Could you check a few things on this model? Use its own coordinates, in mm. A direction names the side the tool comes from. Give positions to 0.01 mm unless a question says otherwise; leave off trailing zeros. Loops run counter-clockwise (first coordinate to the right, second up) from the corner with the lowest first, then second, coordinate; pieces in that order, holes last. Notation, with made-up numbers: (-1, 68) - (48, 68) arc R21 cw to (48, 73) - close; hole circle Ø4 at (-25, 70.25). An arc over 180 degrees is marked (long way). Answer in a Markdown table with one row per item. Add a question column.
```python
from build123d import *

# Parameters (mm, degrees)
SKETCH1_W           = 70
SKETCH1_H           = 60
SKETCH1_R           = 1.5875
SKETCH1_R_2         = 4.499999999
BOSS_EXTRUDE1_DEPTH = 10


with BuildPart() as part:
    # Sketch1 → Boss-Extrude1 (new body)
    with BuildSketch(Plane(origin=(0, 0, 0), x_dir=(0, 0, -1), z_dir=(1, 0, 0))):
        with Locations((3.813160791, 27.897530874)):
            Rectangle(SKETCH1_W, SKETCH1_H)
        with Locations((-16.186839209, 52.897530874)):
            Circle(SKETCH1_R, mode=Mode.SUBTRACT)
        with Locations((-16.186839209, 2.897530874)):
            Circle(SKETCH1_R, mode=Mode.SUBTRACT)
        with Locations((23.813160791, 2.897530874)):
            Circle(SKETCH1_R, mode=Mode.SUBTRACT)
        with Locations((23.813160791, 52.897530874)):
            Circle(SKETCH1_R, mode=Mode.SUBTRACT)
        with Locations((3.813160791, 27.897530874)):
            Circle(SKETCH1_R_2, mode=Mode.SUBTRACT)
        with BuildLine():
            Line((-5.464379102, 30.775341326), (-4.081605515, 33.606305024))
            ThreePointArc((-4.081605515, 33.606305024), (-1.369183898, 34.499769949), (-0.528409533, 31.770555947))
            Line((-0.528409533, 31.770555947), (-1.869576404, 29.020756356))
            ThreePointArc((-1.869576404, 29.020756356), (-4.544523089, 28.10012945), (-5.464379102, 30.775341326))
        make_face(mode=Mode.SUBTRACT)
        with BuildLine():
            Line((5.31316079, 18.397530874), (2.313160791, 18.397530874))
            ThreePointArc((2.313160791, 18.397530874), (0.313160792, 20.397530874), (2.313160791, 22.397530873))
            Line((2.313160791, 22.397530873), (5.31316079, 22.397530873))
            ThreePointArc((5.31316079, 22.397530873), (7.313160789, 20.397530874), (5.31316079, 18.397530874))
        make_face(mode=Mode.SUBTRACT)
        with BuildLine():
            Line((5.31316079, 33.374248764), (2.313160791, 33.374248764))
            ThreePointArc((2.313160791, 33.374248764), (0.31316079, 35.374248765), (2.313160791, 37.374248765))
            Line((2.313160791, 37.374248765), (5.31316079, 37.374248765))
            ThreePointArc((5.31316079, 37.374248765), (7.313160791, 35.374248765), (5.31316079, 33.374248764))
        make_face(mode=Mode.SUBTRACT)
        with BuildLine():
            Line((9.471997672, 29.038205562), (8.081045524, 31.961596177))
            ThreePointArc((8.081045524, 31.961596177), (9.113942414, 34.555839775), (11.733632625, 33.589300054))
            Line((11.733632625, 33.589300054), (13.083423708, 30.758314735))
            ThreePointArc((13.083423708, 30.758314735), (12.137765277, 28.092547131), (9.471997672, 29.038205562))
        make_face(mode=Mode.SUBTRACT)
    extrude(amount=BOSS_EXTRUDE1_DEPTH)


solid = part.part
```
(1) We'd pull the mould along Y, two halves only. Please class faces 1 (the flat face through (0, 35, 4)), 2 (the flat face through (5, -2.102, -3)), 3 (the cylindrical face through (4.93, 34.52, 1.41)): pulls with the +Y half, pulls with the -Y half, needs draft (parallel to the pull), parting line crosses it, or undercut.
(2) Please list where these lines run through material, in increasing order: line 1 (Z direction, x = 1.25, y = 3); line 2 (Y direction, x = 7.5, z = -4); line 3 (Z direction, x = 6.25, y = 1.5).
(3) I want a section at A-A on z = -23. Please give me the cut outline in (x, y).
(4) I want a section at B-B on x = 8.25. State how many separate pieces and enclosed holes the cut face has, then the cut area to 3 significant figures.
(5) On a 3-axis mill with a long thin cutter (end or side, diameter ignored), from which of +Z, -Z, +X, -X, +Y, -Y can I reach the whole of each face in a straight line? I mean faces 4 (the flat face through (10, 35, 4)), 5 (the flat face through (5, 18.398, -4)). Say none if no direction works.
(6) For pin 1 Ø2.5 at (y, z) = (2.9, 16.19) entering from +X, with a flat end and sliding along its axis, tell me the tip position at first contact or that it passes through.
Reported:
| question | item | result |
|---|---|---|
| 1 | face 1 | needs draft |
| 1 | face 2 | pulls with the -Y half |
| 1 | face 3 | undercut |
| 2 | line 1 | -38.81 to -25.4, -22.23 to 14.6, 17.77 to 31.19 |
| 2 | line 2 | -2.1 to 18.4, 22.4 to 23.4, 32.39 to 33.37, 37.37 to 57.9 |
| 2 | line 3 | -38.81 to -24.57, -23.06 to 15.43, 16.94 to 31.19 |
| 3 | outline | (0, -2.1) - (10, -2.1) - (10, 1.53) - (0, 1.53) - close; (0, 4.26) - (10, 4.26) - (10, 51.53) - (0, 51.53) - close; (0, 54.26) - (10, 54.26) - (10, 57.9) - (0, 57.9) - close |
| 4 | separate pieces | 1 |
| 4 | enclosed holes | 9 |
| 4 | area | 4,010 mm² |
| 5 | face 4 | +Z, -Z, +X, +Y, -Y |
| 5 | face 5 | +X, -X |
| 6 | pin 1 | through |
